```python
from build123d import *

# Parameters (mm, degrees)
SKETCH1_W            = 490
SKETCH1_H            = 335.5
BOSS_EXTRUDE1_DEPTH  = 6
SKETCH5_W            = 6
SKETCH5_H            = 77
CUT_EXTRUDE2_DEPTH   = 594.882353669
SKETCH3_W            = 377
SKETCH3_H            = 300
CUT_EXTRUDE3_DEPTH   = 594.882353669
SKETCH6_W            = 157.333333333
SKETCH6_H            = 6
CUT_EXTRUDE4_DEPTH   = 594.882353669
M8_CLEARANCE_SLOT1_D = 8.4


with BuildPart() as part:
    # Sketch1 → Boss-Extrude1 (new body)
    with BuildSketch(Plane.XY):
        with Locations((245, 167.75)):
            Rectangle(SKETCH1_W, SKETCH1_H)
    extrude(amount=BOSS_EXTRUDE1_DEPTH)

    # Sketch5 → Cut-Extrude2 (cut, through all)
    with BuildSketch(Plane.XY.offset(6)):
        with Locations((3, 297)):
            Rectangle(SKETCH5_W, SKETCH5_H)
        with Locations((3, 38.5)):
            Rectangle(SKETCH5_W, SKETCH5_H)
        with Locations((487, 297)):
            Rectangle(SKETCH5_W, SKETCH5_H)
        with Locations((487, 38.5)):
            Rectangle(SKETCH5_W, SKETCH5_H)
    extrude(amount=-CUT_EXTRUDE2_DEPTH, mode=Mode.SUBTRACT)

    # Sketch3 → Cut-Extrude3 (cut, through all)
    with BuildSketch(Plane.XY.offset(6)):
        with Locations((245, 164.75)):
            Rectangle(SKETCH3_W, SKETCH3_H)
    extrude(amount=-CUT_EXTRUDE3_DEPTH, mode=Mode.SUBTRACT)

    # Sketch6 → Cut-Extrude4 (cut, through all)
    with BuildSketch(Plane.XY.offset(6)):
        with Locations((405.333333334, 332.5)):
            Rectangle(SKETCH6_W, SKETCH6_H)
        with Locations((84.666666667, 332.5)):
            Rectangle(SKETCH6_W, SKETCH6_H)
    extrude(amount=-CUT_EXTRUDE4_DEPTH, mode=Mode.SUBTRACT)

    # M8 Clearance Slot1 (through all)
    with Locations(Plane.XY.offset(6)):
        with Locations((36, 167.75), (454, 167.75)):
            Hole(M8_CLEARANCE_SLOT1_D / 2)


solid = part.part
```
Could you check a few things on this model? Use its own coordinates, in mm. Coordinates: 2 decimals unless noted, no trailing zeros. Loops run counter-clockwise (first coordinate to the right, second up) from the corner with the lowest first, then second, coordinate; pieces in that order, holes last.
1) Imagine slicing it at C-C (z = 4.85). List the corners of the cut face in (x, y) for me, and give its area (3 significant figures).
Reported:
outline: (0, 77) - (6, 77) - (6, 0) - (484, 0) - (484, 77) - (490, 77) - (490, 258.5) - (484, 258.5) - (484, 329.5) - (326.67, 329.5) - (326.67, 335.5) - (163.33, 335.5) - (163.33, 329.5) - (6, 329.5) - (6, 258.5) - (0, 258.5) - close; hole circle Ø8.4 at (36, 167.75); hole (56.5, 14.75) - (433.5, 14.75) - (433.5, 314.75) - (56.5, 314.75) - close; hole circle Ø8.4 at (454, 167.75)
area: 47,400 mm2
2) Imagine slicing it at A-A (x = 144.5). List the corners of the cut face in (y, z) for me.
Reported:
outline: (0, 0) - (14.75, 0) - (14.75, 6) - (0, 6) - close; (314.75, 0) - (329.5, 0) - (329.5, 6) - (314.75, 6) - close
3) Imagine slicing it at B-B (y = 97). List the corners of the cut face in (x, z) for me.
Reported:
outline: (0, 0) - (56.5, 0) - (56.5, 6) - (0, 6) - close; (433.5, 0) - (490, 0) - (490, 6) - (433.5, 6) - close
4) Will these pins go through, and if not, where does the flat tip stop? pin 1 Ø3 at (y, z) = (334, 3.5) entering from +X; pin 2 Ø1.8 at (x, z) = (3, 4.5) entering from -Y; pin 3 Ø3 at (x, z) = (412, 2) entering from +Y.
Reported:
pin 1: stops at x = 326.67
pin 2: stops at y = 77
pin 3: stops at y = 329.5
5) Please list where these lines run through material, in increasing order: line 1 along X through (y, z) = (239, 1.35); line 2 along Y through (x, z) = (36, 1.8); line 3 along X through (y, z) = (303, 5.2).
Reported:
line 1: x = 0 to 56.5, 433.5 to 490
line 2: y = 0 to 163.55, 171.95 to 329.5
line 3: x = 6 to 56.5, 433.5 to 484
